For this review, take the finished solid that the model builds, in its own axes (mm). Face numbers are marked on the shaded views. Coordinates: 2 decimals unless noted, no trailing zeros. Loops run counter-clockwise (first coordinate to the right, second up) from the corner with the lowest first, then second, coordinate; pieces in that order, holes last. Notation, with made-up numbers: (47, 38) - (89, 38) arc R28 ccw to (89, 62) - close; hole circle Ø6 at (50, 28). An arc over 180 degrees is marked (long way). Use one line per item in the form item = value. Start each with the question number.
1. Add section B-B on x = -10.5. Give the boundary of the cut face in (y, z), and give its area (3 significant figures).
2. To check wall thickness, follow probe 1 along X at (y, z) = (-56, 0.4); probe 2 along Y at (x, z) = (9.5, 1.65); probe 3 along X at (y, z) = (-10.5, 0.6). State the ranges of each line that lie inside material, in increasing order.
3. Draft analysis for pull direction Z (two halves, no side actions). For the marked faces 1 and 2, state which applies: +Z half, -Z half, draft (parallel to the pull), parting line (faces both ways), or undercut.
4. For pin 1 Ø0.8 at (x, z) = (-0.5, 1) entering from -Y; pin 2 Ø1.2 at (x, z) = (-5.5, 1) entering from -Y; pin 3 Ø1.2 at (y, z) = (-61, 1) entering from -X, all flat-tipped, find the tip position at first contact; note any pin that passes through.
5. Add section A-A on z = 1.9. Give the boundary of the cut face in (x, y).
6. Add section D-D on x = 13. Give the boundary of the cut face in (y, z).
7. Add section C-C on y = -52.5. Give the boundary of the cut face in (x, z).
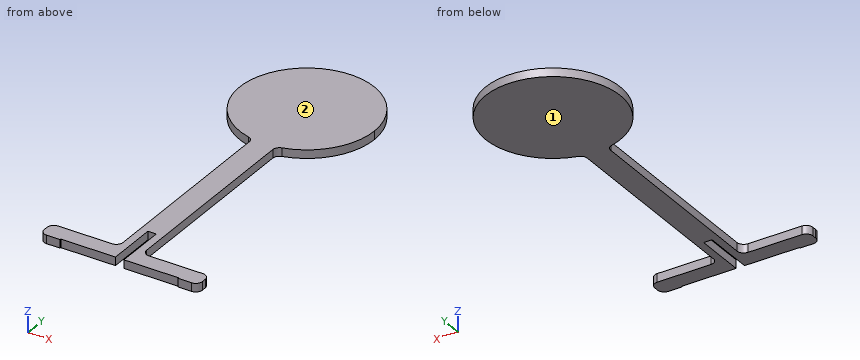
```python
from build123d import *

# Parameters (mm, degrees)
F0_W     = 6
F0_H     = 0.3
F1_DEPTH = 2.5
F2_R     = 2


# Not quite as in the source:
# - a feature names something its author has since deleted; it is built from what else it names


with BuildPart() as f1:
    # F0 (on Top) → F1 (new body)
    with BuildSketch(Plane.XY):
        with BuildLine():
            ThreePointArc((3.5, -3), (0, -3.3086313325), (-3.5, -3))
            Line((-3.5, -3), (-3.5, -65))
            Line((-3.5, -65), (-23.5, -65))
            Line((-23.5, -65), (-23.5, -70))
            Line((-23.5, -70), (-17.5, -70))
            Line((-17.5, -70), (-1.25, -70))
            Line((-1.25, -70), (-1.25, -55))
            Line((-1.25, -55), (1.25, -55))
            Line((1.25, -55), (1.25, -70))
            Line((1.25, -70), (17.5, -70))
            Line((17.5, -70), (23.5, -70))
            Line((23.5, -70), (23.5, -65))
            Line((23.5, -65), (3.5, -65))
            Line((3.5, -65), (3.5, -3))
        make_face()
        with BuildLine():
            ThreePointArc((20, 16.6913686675), (-12.8452325787, 32.0210783843), (-3.5, -3))
            ThreePointArc((-3.5, -3), (0, -3.3086313325), (3.5, -3))
            ThreePointArc((3.5, -3), (15.3297097168, 3.8461360889), (20, 16.6913686675))
        make_face()
        with Locations((-20.5, -70.15)):
            Rectangle(F0_W, F0_H)
        with Locations((20.5, -70.15)):
            Rectangle(F0_W, F0_H)
    extrude(amount=F1_DEPTH)

    # F2
    f2_edges = [f1.edges().sort_by_distance(p)[0] for p in [
        (-3.5, -3, 1.25),
        (3.5, -3, 1.25),
        (23.5, -65, 1.25),
        (-23.5, -65, 1.25),
        (-3.5, -65, 1.25),
        (3.5, -65, 1.25),
        (-23.5, -70.3, 1.25),
        (23.5, -70.3, 1.25),
    ]]
    fillet(f2_edges, radius=F2_R)


solid = f1.part
```
Conclusion:
q1.outline = (-70, 0) - (-65, 0) - (-65, 2.5) - (-70, 2.5) - close; (-0.33, 0) - (33.71, 0) - (33.71, 2.5) - (-0.33, 2.5) - close
q1.area = 97.6 mm^2
q2.probe_1 = -3.5 to -1.25, 1.25 to 3.5
q2.probe_2 = -70 to -65, -0.91 to 34.29
q2.probe_3 = -3.5 to 3.5
q3.face_1 = -Z half
q3.face_2 = +Z half
q4.pin_1 = -55
q4.pin_2 = -70
q4.pin_3 = -3.5
q5.outline = (-23.5, -68.3) arc R2 ccw to (-21.5, -70.3) - (-17.5, -70.3) - (-17.5, -70) - (-1.25, -70) - (-1.25, -55) - (1.25, -55) - (1.25, -70) - (17.5, -70) - (17.5, -70.3) - (21.5, -70.3) arc R2 ccw to (23.5, -68.3) - (23.5, -67) arc R2 ccw to (21.5, -65) - (5.5, -65) arc R2 cw to (3.5, -63) - (3.5, -4.61) arc R2 cw to (5, -2.67) arc R20 ccw (long way) to (-5, -2.67) arc R2 cw to (-3.5, -4.61) - (-3.5, -63) arc R2 cw to (-5.5, -65) - (-21.5, -65) arc R2 ccw to (-23.5, -67) - close
q6.outline = (-70, 0) - (-65, 0) - (-65, 2.5) - (-70, 2.5) - close; (1.49, 0) - (31.89, 0) - (31.89, 2.5) - (1.49, 2.5) - close
q7.outline = (-3.5, 0) - (3.5, 0) - (3.5, 2.5) - (-3.5, 2.5) - close
